Input: part model. Units: mm. Frame: model coordinates. Coordinates: 2 decimals unless noted, no trailing zeros. Loops run counter-clockwise (first coordinate to the right, second up) from the corner with the lowest first, then second, coordinate; pieces in that order, holes last. Notation, with made-up numbers: M 18,-30 L 58,-30 A11 ccw 58,-15 Z; hole C 59.25,18.25 d11. An arc over 180 degrees is marked long. Use a Markdown table: item, result. Add a question column.
1. Pin query (flat end, axial travel): pin 1 (3 mm diameter, centred on x = -7, z = -6, fed in from -Y); pin 2 (5 mm diameter, centred on x = -4.5, y = 16, fed in from -Z); pin 3 (10 mm diameter, centred on y = 2.5, z = 7, fed in from -X). Return the tip coordinate at first contact, or that it passes through.
2. Section B-B on z = 0. Output: boundary loops of the cut face in (x, y), then the cut area to 3 significant figures.
3. Section A-A on x = 0. Output: boundary loops of the cut face in (y, z), then the cut area to 3 significant figures.
4. Line query: L1, parallel to Z at x = 0, y = 11.75; L2, parallel to Z at x = -2.5, y = 5; L3, parallel to X at y = 12, z = 5. Output: solid intervals per line, ascending. Write a range as [from, to].
5. Section C-C on y = 12. Output: boundary loops of the cut face in (x, z).
6. Section D-D on y = 1.75. Output: boundary loops of the cut face in (x, z), then the cut area to 3 significant figures.
7. Draft query along X for faces 1 (the cylindrical face through (-6, 10, -8)), 2 (the cylindrical face through (5.894, 11.269, -0.259)), 3 (the flat face through (-4.3, 20, 4.3)). Return one class per face: +X half, -X half, draft (parallel to the pull), parting line (faces both ways), or undercut.
```python
from build123d import *

# Parameters (mm, degrees)
SKETCH1_R               = 10
BOSS_EXTRUDE1_DEPTH     = 20
CUT_EXTRUDE1_DEPTH      = 25.494897428
CUT_EXTRUDE1_DEPTH_BACK = 25.494897428
SKETCH2_R               = 15
G1_4_TAPPED_HOLE1_D     = 11.8


with BuildPart() as part:
    # Sketch1 → Boss-Extrude1 (new body)
    with BuildSketch(Plane(origin=(0, 0, 0), x_dir=(1, 0, 0), z_dir=(0, 1, 0))):
        with Locations(Location((0, 0, 0), (0, 0, 270))):
            Circle(SKETCH1_R)
    extrude(amount=BOSS_EXTRUDE1_DEPTH)

    # Sketch2 → Cut-Extrude1 (cut, two sides: drawn at the far end of the back side and taken through both)
    with BuildSketch(Plane.XY.offset(-CUT_EXTRUDE1_DEPTH_BACK)):
        with Locations((0, -11)):
            Circle(SKETCH2_R)
    extrude(amount=CUT_EXTRUDE1_DEPTH + CUT_EXTRUDE1_DEPTH_BACK, mode=Mode.SUBTRACT)

    # G1/4 Tapped Hole1 (through all)
    with Locations(Plane(origin=(0, 20, 0), x_dir=(1, 0, 0), z_dir=(0, 1, 0))):
        with Locations((0, 0)):
            Hole(G1_4_TAPPED_HOLE1_D / 2)


solid = part.part
```
Answers below:
| question | item | result |
|---|---|---|
| 1 | pin 1 | stops at y = 1.43 |
| 1 | pin 2 | stops at z = -9.8 |
| 1 | pin 3 | stops at x = -9.8 |
| 2 | outline | M -10,0.18 A15 cw -5.9,2.79 L -5.9,20 L -10,20 Z; M 5.9,2.79 A15 cw 10,0.18 L 10,20 L 5.9,20 Z |
| 2 | area | 151 mm² |
| 3 | outline | M 4,-10 L 20,-10 L 20,-5.9 L 4,-5.9 Z; M 4,5.9 L 20,5.9 L 20,10 L 4,10 Z |
| 3 | area | 131 mm² |
| 4 | L1 | z = [-10, -5.9], [5.9, 10] |
| 4 | L2 | z = [-9.68, -5.34], [5.34, 9.68] |
| 4 | L3 | x = [-8.66, -3.13], [3.13, 8.66] |
| 5 | outline | C 0,0 d20; hole C 0,0 d11.8 |
| 6 | outline | M -7.9,-6.13 L -7.9,6.13 A10 ccw Z; M 7.9,-6.13 A10 ccw 7.9,6.13 Z |
| 6 | area | 35.1 mm² |
| 7 | face 1 | parting line |
| 7 | face 2 | undercut |
| 7 | face 3 | draft |
